Geometry check sheet. Reference: the model listing, model coordinates, mm. Round coordinates to 2 decimals unless told otherwise and drop trailing zeros. Loops run counter-clockwise (first coordinate to the right, second up) from the corner with the lowest first, then second, coordinate; pieces in that order, holes last. Notation, with made-up numbers: (56, 46.5) - (112, 46.5) arc R4 cw to (112, 51.5) - close; hole circle Ø7 at (-24, 61.25). An arc over 180 degrees is marked (long way). Answer in a Markdown table with one row per item. Add a question column.
Autodesk Inventor part; units mm, degrees
ref_plane "YZ Plane" through (0, 0, 0) normal (1, 0, 0) x (0, 1, 0)
ref_plane "XZ Plane" through (0, 0, 0) normal (0, 1, 0) x (-1, 0, 0)
ref_plane "XY Plane" through (0, 0, 0) normal (0, 0, 1) x (1, 0, 0)
sketch "Эскиз1" plane through (0, 0, 0) normal (0, 0, 1) x (1, 0, 0)
  circle A0 centre (0, 0) radius 12.5
  line L0 (0, -12.5) -> (280, -12.5)
  line L1 (280, -12.5) -> (280, 12.5)
  line L2 (280, 12.5) -> (0, 12.5)
  line L3 (0, 12.5) -> (0, -12.5)
  circle A1 centre (280, 0) radius 12.5
  circle A2 centre (0, 0) radius 7
  circle A3 centre (280, 0) radius 7
  circle A4 centre (0, 7) radius 1.5
  circle A5 centre (7, 0) radius 1.5
  circle A6 centre (0, -7) radius 1.5
  circle A7 centre (-7, 0) radius 1.5
  circle A8 centre (0, 0) radius 3
  circle A9 centre (280, 0) radius 3
  circle A10 centre (287, 0) radius 1.5
  circle A11 centre (280, 7) radius 1.5
  circle A12 centre (280, -7) radius 1.5
  circle A13 centre (273, 0) radius 1.5
  line L4 (138, 12.5) -> (142, 12.5)
  line L5 (142, 12.5) -> (142, 0)
  line L6 (142, 0) -> (138, 0)
  line L7 (138, 0) -> (138, 12.5)
  point P0 (280, -12.5)
  point P1 (140, 12.5)
  point P2 (140, 12.5)
  point P3 (142, 12.5)
  dimension "d0" = 25
  dimension "d2" = 14
  dimension "d3" = 14
  dimension "d4" = 3
  dimension "d5" = 3
  dimension "d6" = 3
  dimension "d7" = 3
  dimension "d8" = 6
  dimension "d9" = 6
  dimension "d10" = 3
  dimension "d11" = 3
  dimension "d12" = 3
  dimension "d13" = 3
  dimension "d16" = 0
  dimension "d17" = 4
  dimension "d27" = 280
extrude "Выдавливание1" add sketch "Эскиз1" along normal blind 4 contours A0 L3 A6 A2 A5 A4 | A0 L2 L7 L6 L5 A1 L0 | L3 A4 A2 A7 A6 A0 | A1 L1 A11 A3 A13 A12 | L1 A12 A3 A10 A11 A1 | A4 L3 A8 A6 A2 A7 | A4 A2 A5 A6 L3 A8 | A3 A13 A11 L1 A9 A12 | L1 A9 A11 A3 A10 A12
sketch "Эскиз2" plane through (0, 0, 4) normal (0, 0, 1) x (1, 0, 0)
  line L0 (152, 23.4347) -> (358.3941, 23.4347)
  line L1 (358.3941, 23.4347) -> (358.3941, -33.9487)
  line L2 (358.3941, -33.9487) -> (152, -33.9487)
  line L3 (152, -33.9487) -> (152, 23.4347)
  line L4 (142, 12.5) -> (142, 0)
  point P0 (0, 0)
  dimension "d18" = 10
extrude "Выдавливание2" cut sketch "Эскиз2" against normal blind 10
fillet "Сопряжение1" radius 2 2 edges at (152, 12.5, 2) (152, -12.5, 2)
sketch "Эскиз3" plane through (0, 0, 4) normal (0, 0, 1) x (1, 0, 0)
  line L0 (138, 12.5) -> (0, 12.5)
  line L1 (67, 12.5) -> (71, 12.5)
  line L2 (71, 12.5) -> (71, 0)
  line L3 (71, 0) -> (67, 0)
  line L4 (67, 0) -> (67, 12.5)
  line L5 (142, 0) -> (138, 0)
  point P0 (0, 0)
  point P1 (69, 12.5)
  point P2 (69, 12.5)
  point P3 (71, 12.5)
  point P4 (140, 0)
  dimension "d22" = 0
  dimension "d23" = 4
extrude "Выдавливание3" cut sketch "Эскиз3" against normal blind 10
properties material "Дерево (вишня)"
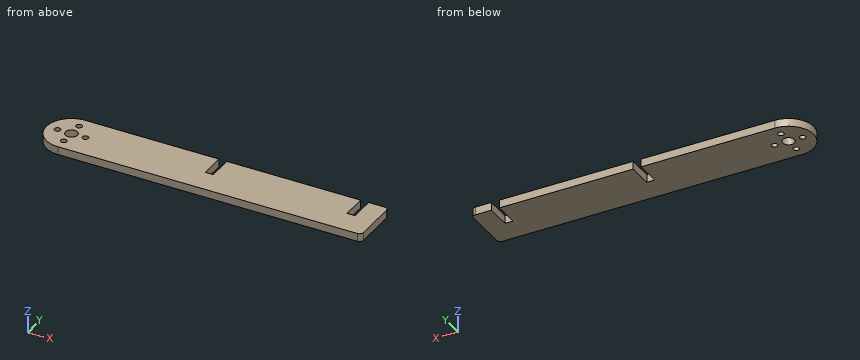
Q1. Cross-section at B-B, the plane z = 1.1. Enter the section's corners in (x, y).
Q2. Cross-section at A-A, the plane x = 7. Enter the section's corners in (y, z).
Q3. Cross-section at C-C, the plane y = 7. Enter the section's corners in (x, z).
Q4. Scan lines: line 1 (Y direction, x = 0, z = 2.3); line 2 (X direction, y = -0.25, z = 1.75); line 3 (X direction, y = 11, z = 1). Record each from-to range of solid material in increasing order. Write a range as from..to.
Q5. Depth check by flat-ended pin: P1, Ø3.5, axis at x = 0, y = 7, coming from the +Z side; P2, Ø2, axis at x = 69, z = 2, coming from the +Y side; P3, Ø1.2, axis at y = 5, z = 1.5, coming from the -X side. Enter the tip coordinate at first touch or a pass-through.
Check sheet entries:
| question | item | result |
|---|---|---|
| 1 | outline | (0, -12.5) - (150, -12.5) arc R2 ccw to (152, -10.5) - (152, 10.5) arc R2 ccw to (150, 12.5) - (142, 12.5) - (142, 0) - (138, 0) - (138, 12.5) - (71, 12.5) - (71, 0) - (67, 0) - (67, 12.5) - (0, 12.5) arc R12.5 ccw to start; hole circle Ø3 at (-7, 0); hole circle Ø6 at (0, 0); hole circle Ø3 at (0, -7); hole circle Ø3 at (0, 7); hole circle Ø3 at (7, 0) |
| 2 | outline | (-12.5, 0) - (-1.5, 0) - (-1.5, 4) - (-12.5, 4) - close; (1.5, 0) - (12.5, 0) - (12.5, 4) - (1.5, 4) - close |
| 3 | outline | (-10.36, 0) - (-1.5, 0) - (-1.5, 4) - (-10.36, 4) - close; (1.5, 0) - (67, 0) - (67, 4) - (1.5, 4) - close; (71, 0) - (138, 0) - (138, 4) - (71, 4) - close; (142, 0) - (152, 0) - (152, 4) - (142, 4) - close |
| 4 | line 1 | -12.5..-8.5, -5.5..-3, 3..5.5, 8.5..12.5 |
| 4 | line 2 | -12.5..-8.48, -5.52..-2.99, 2.99..5.52, 8.48..152 |
| 4 | line 3 | -5.94..67, 71..138, 142..151.94 |
| 5 | P1 | z = 4 |
| 5 | P2 | y = 0 |
| 5 | P3 | x = -11.7 |
